from build123d import *

# Parameters (mm, degrees)
SKETCH026_W     = 140
SKETCH026_H     = 20
PAD024_DEPTH    = 5
SKETCH027_W     = 90
SKETCH027_H     = 10
PAD025_DEPTH    = 20
SKETCH028_R     = 2.7
POCKET002_DEPTH = 5.001


with BuildPart() as part:
    # Sketch026 → Pad024 (new body)
    with BuildSketch(Plane.XY):
        with Locations((70, 10)):
            Rectangle(SKETCH026_W, SKETCH026_H)
    extrude(amount=PAD024_DEPTH)

    # Sketch027 (on Face5 of Pad024) → Pad025 (join)
    with BuildSketch(Plane(origin=(0, 0, 0), x_dir=(1, 0, 0), z_dir=(0, 0, -1))):
        Polygon((20, 0), (25, 0), (115, 0), (120, 0), (120, -20), (115, -20), (25, -20), (20, -20), align=None)
        with Locations((70, -10)):
            Rectangle(SKETCH027_W, SKETCH027_H, mode=Mode.SUBTRACT)
    extrude(amount=PAD025_DEPTH)

    # Sketch028 (on Face4 of Pad025) → Pocket002 (cut, through all)
    with BuildSketch(Plane(origin=(0, 0, 0), x_dir=(1, 0, 0), z_dir=(0, 0, -1))):
        with Locations((10, -10)):
            Circle(SKETCH028_R)
        with Locations((130, -10)):
            Circle(SKETCH028_R)
    extrude(amount=-POCKET002_DEPTH, mode=Mode.SUBTRACT)


solid = part.part
Design review of the part built by this model. Coordinates are the model's own, in mm. A direction names the side the tool comes from. Round coordinates to 2 decimals unless told otherwise and drop trailing zeros. Order: outer loops, then holes, each group sorted by start corner. A loop starts at its lowest first (then second) coordinate and runs counter-clockwise, first axis right, second up.
1) Consider section D-D (y = 1.5). State the section outline as (x, z) points, plus the area to 3 significant figures.
The answers:
outline: (0, 0) - (20, 0) - (20, -20) - (120, -20) - (120, 0) - (140, 0) - (140, 5) - (0, 5) - close
area: 2,700 mm2
2) Clearance check with flat-ended pins moving along their axes: pin 1 Ø6 at (y, z) = (8.5, -9) entering from -X; pin 2 Ø10 at (y, z) = (6, -16) entering from +X; pin 3 Ø3 at (x, y) = (55, 9.5) entering from -Z. State where each tip first meets the part, or that it passes through.
The answers:
pin 1: stops at x = 20
pin 2: stops at x = 120
pin 3: stops at z = 0
3) Consider section C-C (z = 3). State the section outline as (x, y) points, plus the area to 3 significant figures.
The answers:
outline: (0, 0) - (140, 0) - (140, 20) - (0, 20) - close; hole circle Ø5.4 at (10, 10); hole circle Ø5.4 at (130, 10)
area: 2,750 mm2
4) Consider section B-B (z = -15.5). State the section outline as (x, y) points.
The answers:
outline: (20, 0) - (120, 0) - (120, 20) - (20, 20) - close; hole (25, 5) - (115, 5) - (115, 15) - (25, 15) - close
5) Draft analysis for pull direction Y (two halves, no side actions). For faces 4 (the flat face through (115, 10, -10)), 5 (the flat face through (71, 3, -20)), 6 (the flat face through (69, 20, -8)), state which applies: released by +Y, released by -Y, zero draft, split by the parting line, or undercut.
The answers:
face 4: undercut
face 5: zero draft
face 6: released by +Y
6) Machinability: for faces 1 (the flat face through (12.1, 12.4, 0)), 2 (the flat face through (127.6, 12.4, 0)), 3 (the flat face through (69, 15, -10)), which of the approach directions +Z, -Z, +X, -X, +Y, -Y give a long, thin tool a straight path to every point of the face, cutting with its end or side? Answer none if there is none.
The answers:
face 1: -Z, -X, +Y, -Y
face 2: -Z, +X, +Y, -Y
face 3: -Z
7) Consider section A-A (x = 10). State the section outline as (y, z) points, plus the area to 3 significant figures.
The answers:
outline: (0, 0) - (7.3, 0) - (7.3, 5) - (0, 5) - close; (12.7, 0) - (20, 0) - (20, 5) - (12.7, 5) - close
area: 73.0 mm2
8) For L1, parallel to X at y = 10, z = 2.85; L2, parallel to X at y = 6.25, z = -2.25; L3, parallel to Y at x = 63, z = -14.25, list the stretches that pass through material, from the lowest coordinate up.
The answers:
L1: x = 0 to 7.3, 12.7 to 127.3, 132.7 to 140
L2: x = 20 to 25, 115 to 120
L3: y = 0 to 5, 15 to 20
